Model file for the job. Use its own axes, mm. Face numbers are marked on the shaded views. Round coordinates to 2 decimals unless told otherwise and drop trailing zeros. Loops run counter-clockwise (first coordinate to the right, second up) from the corner with the lowest first, then second, coordinate; pieces in that order, holes last. Notation, with made-up numbers: (28.5, -30) - (49.5, -30) arc R26 cw to (49.5, -3) - close; hole circle Ø6 at (49.5, -26.75). An arc over 180 degrees is marked (long way). Answer as a JSON object with one key per item and string values.
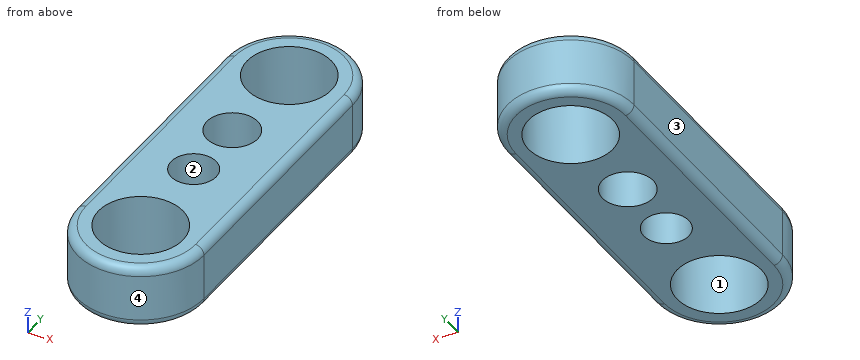
from build123d import *

# Parameters (mm, degrees)
BOSS_EXTRUDE2_DEPTH = 19.05
SKETCH2_R           = 12.7
CUT_EXTRUDE1_DEPTH  = 76.815021516
FILLET1_R           = 2.54
FILLET2_R           = 2.54
SKETCH9_R           = 7.651092206
SKETCH9_R_2         = 6.766631781
CUT_EXTRUDE7_DEPTH  = 76.815021516


with BuildPart() as part:
    # Sketch1 → Boss-Extrude2 (new body)
    with BuildSketch(Plane.XY):
        with BuildLine():
            Line((-29.739928058, 28.163848921), (-29.739928058, -48.036151079))
            ThreePointArc((-29.739928058, -48.036151079), (-10.689928058, -67.086151079), (8.360071942, -48.036151079))
            Line((8.360071942, -48.036151079), (8.360071942, 28.163848921))
            ThreePointArc((8.360071942, 28.163848921), (-10.689928058, 47.213848921), (-29.739928058, 28.163848921))
        make_face()
    extrude(amount=BOSS_EXTRUDE2_DEPTH)

    # Sketch2 → Cut-Extrude1 (cut, through all)
    with BuildSketch(Plane(origin=(0, 0, 0), x_dir=(-1, 0, 0), z_dir=(0, 0, -1))):
        with Locations((10.689928058, 28.163848921)):
            Circle(SKETCH2_R)
        with Locations((10.689928058, -48.036151079)):
            Circle(SKETCH2_R)
    extrude(amount=-CUT_EXTRUDE1_DEPTH, mode=Mode.SUBTRACT)

    # Fillet1
    fillet1_edges = [part.edges().sort_by_distance(p)[0] for p in [
        (8.360071942, -9.936151079, 19.05),
        (-10.689928058, 47.213848921, 19.05),
        (-29.739928058, -9.936151079, 19.05),
        (-10.689928058, -67.086151079, 19.05),
    ]]
    fillet(fillet1_edges, radius=FILLET1_R)

    # Fillet2
    fillet2_edges = [part.edges().sort_by_distance(p)[0] for p in [
        (-10.689928058, 47.213848921, 0),
        (8.360071942, -9.936151079, 0),
        (-10.689928058, -67.086151079, 0),
        (-29.739928058, -9.936151079, 0),
    ]]
    fillet(fillet2_edges, radius=FILLET2_R)

    # Sketch9 → Cut-Extrude7 (cut, through all)
    with BuildSketch(Plane.XY.offset(19.05)):
        with Locations((-11.320081568, 0)):
            Circle(SKETCH9_R)
        with Locations((-11.320081568, -19.793552428)):
            Circle(SKETCH9_R_2)
    extrude(amount=-CUT_EXTRUDE7_DEPTH, mode=Mode.SUBTRACT)


solid = part.part
1) Slice it at C-C on y = -23. List the corners of the cut face in (x, z).
Values follow:
{"outline": "(-29.74, 2.54) arc R2.54 ccw to (-27.2, 0) - (-17.28, 0) - (-17.28, 19.05) - (-27.2, 19.05) arc R2.54 ccw to (-29.74, 16.51) - close; (-5.36, 0) - (5.82, 0) arc R2.54 ccw to (8.36, 2.54) - (8.36, 16.51) arc R2.54 ccw to (5.82, 19.05) - (-5.36, 19.05) - close"}
2) Two-plate mould, pull along X, no slides. Class the marked faces 1, 2, 3 and 4: pulls with the +X half, pulls with the -X half, needs draft (parallel to the pull), parting line crosses it, or undercut.
Values follow:
{"face 1": "undercut", "face 2": "undercut", "face 3": "pulls with the -X half", "face 4": "parting line crosses it"}
3) Probe probe 1 along Y at (x, z) = (-16, 2.5); probe 2 along Y at (x, z) = (-9, 11.5); probe 3 along Y at (x, z) = (-2, 16.5). List the from-to ranges inside material, lowest first.
Values follow:
{"probe 1": "-66.33 to -59.57, -36.5 to -24.68, -14.91 to -6.05, 6.05 to 16.63, 39.7 to 46.46", "probe 2": "-67.01 to -60.62, -35.45 to -26.15, -13.44 to -7.29, 7.29 to 15.58, 40.75 to 47.14", "probe 3": "-64.99 to -57.3, -38.77 to 18.9, 37.43 to 45.12"}
4) Slice it at D-D on x = -8.5. Count the separate pieces of the cut face and the enclosed holes in it, then the cut area to 3 significant figures.
Values follow:
{"separate pieces": "5", "enclosed holes": "0", "area": "708 mm²"}
5) Drop flat-ended pins along their axis: P1, Ø1, axis at x = -24, z = 9, coming from the -Y side; P2, Ø8, axis at x = 2.5, z = 2, coming from the -Y side; P3, Ø8, axis at x = -20, z = 4.5, coming from the -Y side. Give the stop position or say it passes through.
Values follow:
{"P1": "y = -62.14", "P2": "y = -64.71", "P3": "y = -66.33"}
6) Slice it at B-B on z = 8.5. List the corners of the cut face in (x, y).
Values follow:
{"outline": "(-29.74, -48.04) arc R19.05 ccw to (8.36, -48.04) - (8.36, 28.16) arc R19.05 ccw to (-29.74, 28.16) - close; hole circle Ø25.4 at (-10.69, -48.04); hole circle Ø25.4 at (-10.69, 28.16); hole circle Ø15.3 at (-11.32, 0); hole circle Ø13.53 at (-11.32, -19.79)"}
7) Slice it at A-A on y = 0. List the corners of the cut face in (x, z), then the cut area to 3 significant figures.
Values follow:
{"outline": "(-29.74, 2.54) arc R2.54 ccw to (-27.2, 0) - (-18.97, 0) - (-18.97, 19.05) - (-27.2, 19.05) arc R2.54 ccw to (-29.74, 16.51) - close; (-3.67, 0) - (5.82, 0) arc R2.54 ccw to (8.36, 2.54) - (8.36, 16.51) arc R2.54 ccw to (5.82, 19.05) - (-3.67, 19.05) - close", "area": "429 mm²"}
